Work out the finished part from the listing and answer in its coordinate system (mm). A direction names the side the tool comes from. Round coordinates to 2 decimals unless told otherwise and drop trailing zeros. Loops run counter-clockwise (first coordinate to the right, second up) from the corner with the lowest first, then second, coordinate; pieces in that order, holes last. Notation, with made-up numbers: (77, 81.5) - (107, 81.5) arc R35 cw to (107, 119.5) - close; hole circle Ø4 at (-7.5, 38.5). An arc over 180 degrees is marked (long way). Answer as CSV lines item,"result". Start each with the question number.
Q1. Section B-B on z = 11.5 is taken. Write down the section's boundary in (x, y), then the cut area to 3 significant figures.
Q2. Section C-C on x = 19 is taken. Write down the section's boundary in (y, z).
Q3. Section D-D on y = 20 is taken. Write down the section's boundary in (x, z), then the cut area to 3 significant figures.
Q4. For faces 1 (the face through (-47, -12, 25.183)), 2 (the face through (67, 4.112, 10)), 3 (the face through (-34.951, 11, 29)), determine the directions among +Z, -Z, +X, -X, +Y, -Y from which every point of the face is accessible in a straight line to the end or side of a thin tool.
Q5. Each of these flat-tipped pins is pushed along its axis until it touches: pin 1 Ø12 at (x, y) = (-35, 7) entering from -Z; pin 2 Ø12 at (x, y) = (13, 13) entering from +Z; pin 3 Ø15.5 at (y, z) = (-9.5, 11) entering from +X; pin 4 Ø5.5 at (x, z) = (-43, 33) entering from -Y. Where does it stop, or does it pass through?
Q6. The mould has two halves that part along Y. Classify faces 4 (the face through (17.98, 8.85, 9.52)), 5 (the face through (-60.351, 7, 17)), 6 (the face through (-47, 28.61, 22)): +Y half, -Y half, draft (parallel to the pull), parting line (faces both ways), or undercut.
Q7. Section A-A on y = 0 is taken. Write down the section's boundary in (x, z), then the cut area to 3 significant figures.
Q8. Straight lines are drawn through the part: L1, parallel to Z at x = 38, y = 5; L2, parallel to X at y = -18.5, z = 12.5; L3, parallel to X at y = 1, z = 3.5. For each, find the intervals that lie inside material, in ascending order. Write a range as [from, to].
```python
from build123d import *

# Parameters (mm, degrees)
F0_W     = 94.572848
F0_H     = 56.195463
F0_R     = 10.49808
F1_DEPTH = 19.304
F2_W     = 23.812594
F2_H     = 18.846037
F3_DEPTH = 25.4
F4_W     = 24.497905
F4_H     = 19.304
F5_DEPTH = 14.732


with BuildPart() as f1:
    # F0 (on Top) → F1 (new body)
    with BuildSketch(Plane.XY):
        with Locations((12.33559, 0.512037)):
            Rectangle(F0_W, F0_H)
        with Locations((12.33559, 0)):
            Circle(F0_R, mode=Mode.SUBTRACT)
    extrude(amount=F1_DEPTH)

    # F2 (on face) → F3 (join)
    with BuildSketch(Plane(origin=(-34.950834, 0, 0), x_dir=(0, -1, 0), z_dir=(-1, 0, 0))):
        with Locations((-16.703471, 34.606232)):
            Rectangle(F2_W, F2_H)
        Polygon((-4.797174, 25.183214), (-28.609768, 25.183214), (-28.609768, 0), (27.585695, 0), (27.585695, 25.183214), align=None)
    extrude(amount=F3_DEPTH)

    # F4 (on face) → F5 (join)
    with BuildSketch(Plane.YZ.offset(59.622014)):
        with Locations((16.360816, 9.652)):
            Rectangle(F4_W, F4_H)
    extrude(amount=F5_DEPTH)


solid = f1.part
```
Findings:
1,outline,"(-60.35, -27.59) - (59.62, -27.59) - (59.62, 4.11) - (74.35, 4.11) - (74.35, 28.61) - (-60.35, 28.61) - close; hole circle Ø21 at (12.34, 0)"
1,area,"6,760 mm^2"
2,outline,"(-27.59, 0) - (-8.11, 0) - (-8.11, 19.3) - (-27.59, 19.3) - close; (8.11, 0) - (28.61, 0) - (28.61, 19.3) - (8.11, 19.3) - close"
3,outline,"(-60.35, 0) - (74.35, 0) - (74.35, 19.3) - (-34.95, 19.3) - (-34.95, 44.03) - (-60.35, 44.03) - close"
3,area,"3,230 mm^2"
4,face 1,"+Z, +X, -X, -Y"
4,face 2,"+Z, -Z, +X, -Y"
4,face 3,"+Z, +X, +Y, -Y"
5,pin 1,"stops at z = 0"
5,pin 2,"stops at z = 19.3"
5,pin 3,"stops at x = 59.62"
5,pin 4,"stops at y = 4.8"
6,face 4,"undercut"
6,face 5,"draft"
6,face 6,"+Y half"
7,outline,"(-60.35, 0) - (1.84, 0) - (1.84, 19.3) - (-34.95, 19.3) - (-34.95, 25.18) - (-60.35, 25.18) - close; (22.83, 0) - (59.62, 0) - (59.62, 19.3) - (22.83, 19.3) - close"
7,area,"2,060 mm^2"
8,L1,"z = [0, 19.3]"
8,L2,"x = [-60.35, 59.62]"
8,L3,"x = [-60.35, 1.89], [22.79, 59.62]"
